Could you check a few things on this model? Use its own coordinates, in mm. Face numbers are marked on the shaded views. Give positions to 0.01 mm unless a question says otherwise; leave off trailing zeros. Write each loop counter-clockwise with the first axis right and the second up, starting at its lowest first coordinate (ties: lowest second). Pieces come first, ordered by that corner, then holes. Notation, with made-up numbers: (70, 70) - (101, 70) arc R7 cw to (101, 83) - close; hole circle Ø6 at (-34, 50). An arc over 180 degrees is marked (long way). Answer as CSV lines item,"result". Start each with the question number.
Q1. Will this pin go through, and if not, where does the flat tip stop? pin 1 Ø3 at (x, z) = (-33.5, -4) entering from +Y.
Q2. Imagine slicing it at A-A on x = -6.5. List the corners of the cut face in (y, z) for me.
Q3. Imagine slicing it at C-C on y = 2. List the corners of the cut face in (x, z) for me, and give its area (3 significant figures).
Q4. Imagine slicing it at B-B on z = -4. List the corners of the cut face in (x, y) for me.
Q5. If I drill on line 1 along Z through (x, y) = (-33.5, 1.2); line 2 along X through (y, z) = (1.1, -3.5); line 3 along X through (y, z) = (2.1, -2.25), over which ranges is the centre line in solid material (lowest first)?
Q6. We'd pull the mould along X, two halves only. Please class the marked faces 1, 2 and 3: pulls with the +X half, pulls with the -X half, needs draft (parallel to the pull), parting line crosses it, or undercut.
Autodesk Inventor part; units mm, degrees
ref_plane "YZ Plane" through (0, 0, 0) normal (1, 0, 0) x (0, 1, 0)
ref_plane "XZ Plane" through (0, 0, 0) normal (0, 1, 0) x (-1, 0, 0)
ref_plane "XY Plane" through (0, 0, 0) normal (0, 0, 1) x (1, 0, 0)
sketch "Esquisse1" plane through (0, 0, 0) normal (0, 1, 0) x (-1, 0, 0)
  line L0 (0, 0) -> (40, 0)
  line L1 (40, 0) -> (40, -8)
  line L2 (40, -8) -> (0, -8)
  line L3 (0, -8) -> (0, 0)
  line L4 (40, -4) -> (0, -4) construction
  line L5 (20, 0) -> (20, -8) construction
  circle A0 centre (33.5, -4) radius 2
  circle A1 centre (6.5, -4) radius 2
  dimension "d0" = 8
  dimension "d1" = 40
  dimension "d2" = 27
  dimension "d3" = 4
extrude "Extrusion1" add sketch "Esquisse1" along normal blind 3
fillet "Congé1" radius 2 4 edges at (0, 1.5, 0) (0, 1.5, -8) (-40, 1.5, -8) (-40, 1.5, 0)
properties part number "cell"
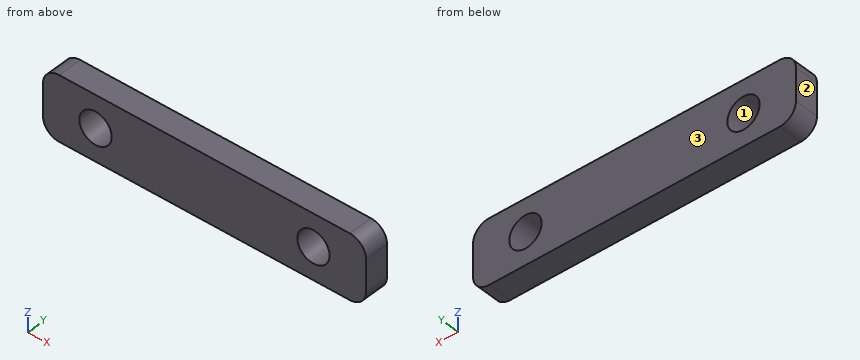
Conclusion:
1,pin 1,"through"
2,outline,"(0, -8) - (3, -8) - (3, -6) - (0, -6) - close; (0, -2) - (3, -2) - (3, 0) - (0, 0) - close"
3,outline,"(-40, -6) arc R2 ccw to (-38, -8) - (-2, -8) arc R2 ccw to (0, -6) - (0, -2) arc R2 ccw to (-2, 0) - (-38, 0) arc R2 ccw to (-40, -2) - close; hole circle Ø4 at (-33.5, -4); hole circle Ø4 at (-6.5, -4)"
3,area,"291 mm^2"
4,outline,"(-40, 0) - (-35.5, 0) - (-35.5, 3) - (-40, 3) - close; (-31.5, 0) - (-8.5, 0) - (-8.5, 3) - (-31.5, 3) - close; (-4.5, 0) - (0, 0) - (0, 3) - (-4.5, 3) - close"
5,line 1,"-8 to -6, -2 to 0"
5,line 2,"-40 to -35.44, -31.56 to -8.44, -4.56 to 0"
5,line 3,"-40 to -34.47, -32.53 to -7.47, -5.53 to 0"
6,face 1,"undercut"
6,face 2,"pulls with the -X half"
6,face 3,"needs draft"
